Autodesk Inventor part; units mm, degrees
ref_plane "YZ Plane" through (0, 0, 0) normal (1, 0, 0) x (0, 1, 0)
ref_plane "XZ Plane" through (0, 0, 0) normal (0, 1, 0) x (-1, 0, 0)
ref_plane "XY Plane" through (0, 0, 0) normal (0, 0, 1) x (1, 0, 0)
sketch "Sketch1" plane through (0, 0, 0) normal (0, 0, 1) x (1, 0, 0)
  line L0 (0, 20.1746) -> (0, -21.4461) construction
  line L1 (-20.2028, 0) -> (20.1685, 0) construction
  line L2 (-12.5, 25) -> (12.5, 25)
  line L3 (12.5, 25) -> (12.5, -25)
  line L4 (12.5, -25) -> (-12.5, -25)
  line L5 (-12.5, -25) -> (-12.5, 25)
  point P0 (0, 0)
  dimension "d0" = 50
  dimension "d1" = 25
  dimension "d2" = 25
  dimension "d3" = 12.5
extrude "Extrusion1" add sketch "Sketch1" along normal blind 1
fillet "Fillet1" radius 5 4 edges at (12.5, 25, 0.5) (-12.5, 25, 0.5) (12.5, -25, 0.5) (-12.5, -25, 0.5)
chamfer "Chamfer1" [suppressed]
equation "\"d0\" = height"
equation "\"d1\" = 0.5 * height"
equation "\"d2\" = width"
equation "\"d3\" = 0.5 * width"
equation "\"d4\" = thickness"
equation "\"d6\" = fillet"
equation "\"fillet\" = 5"
equation "\"chamfer\" = 0"
equation "\"thickness\" = 1"
equation "\"width\" = 25"
equation "\"height\" = 50"
properties part number "Placa Esquinas empalmadas (mm) 25 x 50 x 1" material "Acero, suave"
Work out the finished part from the listing and answer in its coordinate system (mm). Round coordinates to 2 decimals unless told otherwise and drop trailing zeros. Loops run counter-clockwise (first coordinate to the right, second up) from the corner with the lowest first, then second, coordinate; pieces in that order, holes last. Notation, with made-up numbers: M 27.5,-24 L 75.5,-24 A18 ccw 75.5,-1 Z; hole C -13.5,-20.75 d9. An arc over 180 degrees is marked long. One line per question, with ' | ' between items. Start each with the question number.
(1) A flat-ended cylindrical pin translates along its axis: pin 1 Ø4 at (x, y) = (-9, 14.5) entering from -Z. Find the tip coordinate at first contact, or state that the pin passes through.
(2) Find the intervals of material crossed by line 1 (X direction, y = 22, z = 0.35); line 2 (X direction, y = 23.5, z = 0.95); line 3 (Y direction, x = -10.75, z = 0.4), in increasing order.
(3) A cutting plane is placed at A-A on z = 0.25. Write down the section's boundary in (x, y), plus the area to 3 significant figures.
Geometry check:
1) pin 1: stops at z = 0
2) line 1: x = -12.08 to 12.08 | line 2: x = -11.07 to 11.07 | line 3: y = -23.8 to 23.8
3) outline: M -12.5,-20 A5 ccw -7.5,-25 L 7.5,-25 A5 ccw 12.5,-20 L 12.5,20 A5 ccw 7.5,25 L -7.5,25 A5 ccw -12.5,20 Z | area: 1,230 mm²
